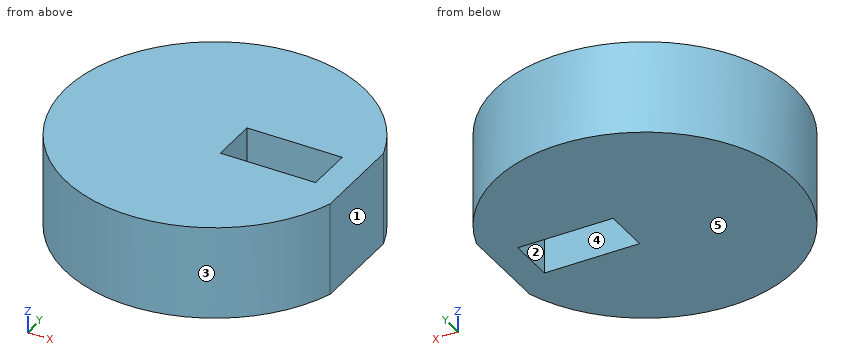
from build123d import *

# Parameters (mm, degrees)
F0_R     = 50.8
F1_DEPTH = 15.875
F2_W     = 2.544178
F2_H     = 31.75
F3_DEPTH = 31.75
F4_W     = 32.380822
F4_H     = 15.875
F5_DEPTH = 31.75


with BuildPart() as f1:
    # F0 (on Top) → F1 (new body, symmetric)
    with BuildSketch(Plane.XY):
        Circle(F0_R)
    extrude(amount=F1_DEPTH, both=True)

    # F2 (on face) → F3 (cut, through all)
    with BuildSketch(Plane.XY.offset(15.875)):
        with Locations((49.527911, 0)):
            Rectangle(F2_W, F2_H)
    extrude(amount=-F3_DEPTH, mode=Mode.SUBTRACT)

    # F4 (on face) → F5 (cut, through all)
    with BuildSketch(Plane.XY.offset(15.875)):
        with Locations((22.540411, 0)):
            Rectangle(F4_W, F4_H)
    extrude(amount=-F5_DEPTH, mode=Mode.SUBTRACT)


solid = f1.part
Design review of the part built by this model. Coordinates are the model's own, in mm. Face numbers are marked on the shaded views. A direction names the side the tool comes from. Coordinates: 2 decimals unless noted, no trailing zeros. Order: outer loops, then holes, each group sorted by start corner. A loop starts at its lowest first (then second) coordinate and runs counter-clockwise, first axis right, second up. Notation, with made-up numbers: M 63,19.5 L 76,19.5 A25 cw 76,46.5 Z; hole C -0.75,-35 d4. An arc over 180 degrees is marked long. Use a Markdown table: item, result.
(1) Draft analysis for pull direction Y (two halves, no side actions). For the marked faces 3, 4 and 5, state which applies: released by +Y, released by -Y, zero draft, split by the parting line, or undercut.
Worked answers:
| item | result |
|---|---|
| face 3 | split by the parting line |
| face 4 | undercut |
| face 5 | zero draft |
(2) For the marked faces 1 and 2, list the 3-axis set-ups (+Z, -Z, +X, -X, +Y, -Y) from which the entire face can be reached by the end or side of a thin tool; tool diameter is ignored.
Worked answers:
| item | result |
|---|---|
| face 1 | +Z, -Z, +X, +Y, -Y |
| face 2 | +Z, -Z |
(3) Add section D-D (y = -33). Give the boundary of the cut face in (x, z) (3 decimals).
Worked answers:
| item | result |
|---|---|
| outline | M -38.622,-15.875 L 38.622,-15.875 L 38.622,15.875 L -38.622,15.875 Z |
(4) Wall thickness on probe 1 along X at (y, z) = (-1, 4); probe 2 along Y at (x, z) = (15, -5); probe 3 along X at (y, z) = (-2.5, -2): over which ranges is each line inside the solid? List them lowest first.
Worked answers:
| item | result |
|---|---|
| probe 1 | x = -50.79 to 6.35, 38.73 to 48.26 |
| probe 2 | y = -48.53 to -7.94, 7.94 to 48.53 |
| probe 3 | x = -50.74 to 6.35, 38.73 to 48.26 |
(5) Add section B-B (x = 24.5). Give the boundary of the cut face in (y, z) (1 decimal), then the cut area to 3 significant figures.
Worked answers:
| item | result |
|---|---|
| outline | M -44.5,-15.9 L -7.9,-15.9 L -7.9,15.9 L -44.5,15.9 Z; M 7.9,-15.9 L 44.5,-15.9 L 44.5,15.9 L 7.9,15.9 Z |
| area | 2,320 mm2 |
(6) Add section A-A (y = 0). Give the boundary of the cut face in (x, z) (3 decimals).
Worked answers:
| item | result |
|---|---|
| outline | M -50.8,-15.875 L 6.35,-15.875 L 6.35,15.875 L -50.8,15.875 Z; M 38.731,-15.875 L 48.256,-15.875 L 48.256,15.875 L 38.731,15.875 Z |
(7) For P1, Ø16, axis at x = 15.5, z = -4, coming from the -Y side; P2, Ø10, axis at y = 33.5, z = -8.5, coming from the -X side; P3, Ø5, axis at y = -15, z = -7, coming from the -X side, all flat-tipped, find the tip position at first contact; note any pin that passes through.
Worked answers:
| item | result |
|---|---|
| P1 | stops at y = -50.24 |
| P2 | stops at x = -42.05 |
| P3 | stops at x = -49.24 |
